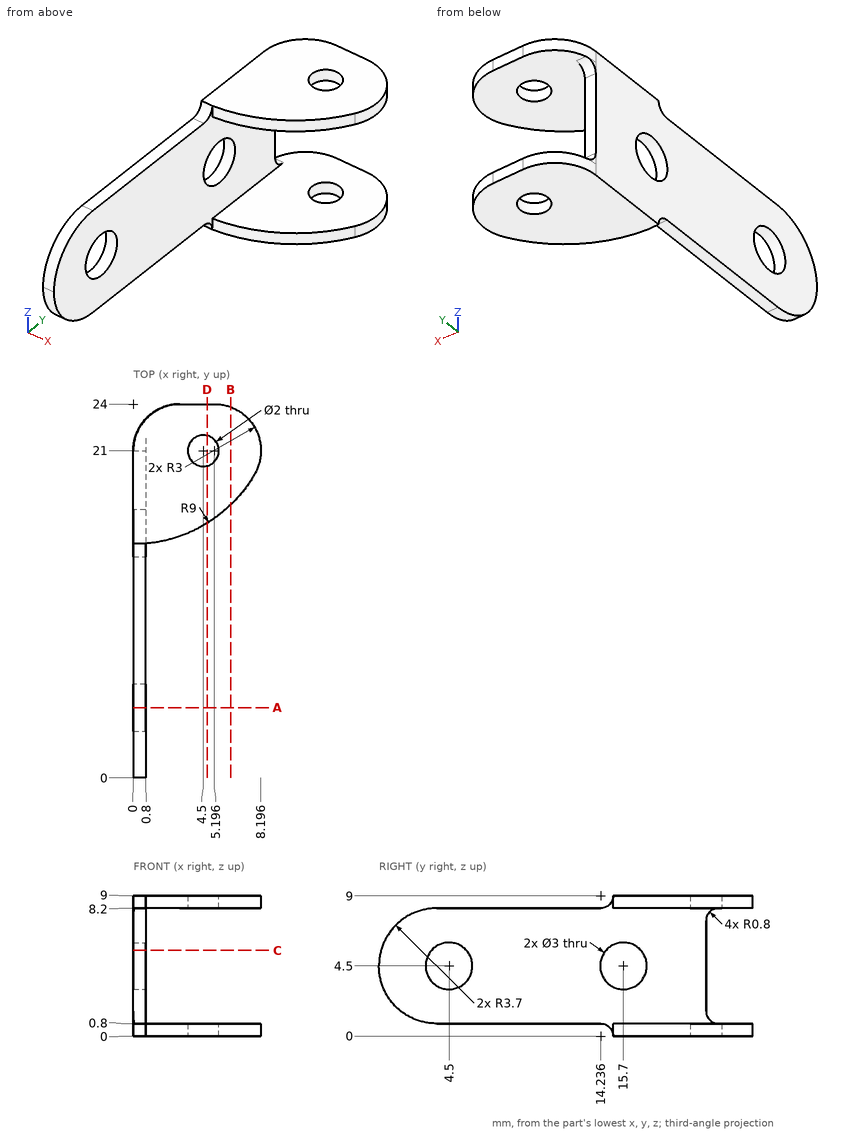
Here's the drawing with two shaded views (mm, measured from the low corner). I have some questions. Coordinates: 2 decimals unless noted, no trailing zeros. Order: outer loops, then holes, each group sorted by start corner. A loop starts at its lowest first (then second) coordinate and runs counter-clockwise, first axis right, second up. Notation, with made-up numbers: (-14, -12) - (22, -12) arc R14 ccw to (22, 5) - close; hole circle Ø8 at (38.25, -13). An arc over 180 degrees is marked (long way). Answer in a Markdown table with one row per item. Add a question column.
(1) If we section it at C-C, the plane z = 5.5: Please give me the cut outline in (x, y).
(2) I need wall thicknesses on L1, parallel to Z at x = 0.5, y = 15.7; L2, parallel to Z at x = 5.75, y = 20.25; L3, parallel to X at y = 14, z = 5. Which ranges of each line are inside material? Lowest first, please.
(3) Will this pin go through, and if not, where does the flat tip stop? pin 1 (1.8 mm diameter, centred on y = 15.7, z = 4.5, fed in from +X).
(4) If we section it at A-A, the plane y = 4.5: Please give me the cut outline in (x, z).
(5) If we section it at B-B, the plane x = 6.25: Please give me the cut outline in (y, z).
(6) If we section it at D-D, the plane x = 4.75: Please give me the cut outline in (y, z) (1 decimal).
Results are:
| question | item | result |
|---|---|---|
| 1 | outline | (0, 0.14) - (0.8, 0.14) - (0.8, 3.38) - (0, 3.38) - close; (0, 5.62) - (0.8, 5.62) - (0.8, 14.58) - (0, 14.58) - close; (0, 16.82) - (0.8, 16.82) - (0.8, 21) - (0, 21) - close |
| 2 | L1 | z = 0 to 3, 6 to 9 |
| 2 | L2 | z = 0 to 0.8, 8.2 to 9 |
| 2 | L3 | x = 0 to 0.8 |
| 3 | pin 1 | passes through |
| 4 | outline | (0, 0.8) - (0.8, 0.8) - (0.8, 3) - (0, 3) - close; (0, 6) - (0.8, 6) - (0.8, 8.2) - (0, 8.2) - close |
| 5 | outline | (17.52, 0) - (23.81, 0) - (23.81, 0.8) - (17.52, 0.8) - close; (17.52, 8.2) - (23.81, 8.2) - (23.81, 9) - (17.52, 9) - close |
| 6 | outline | (16.4, 0) - (20, 0) - (20, 0.8) - (16.4, 0.8) - close; (16.4, 8.2) - (20, 8.2) - (20, 9) - (16.4, 9) - close; (22, 0) - (24, 0) - (24, 0.8) - (22, 0.8) - close; (22, 8.2) - (24, 8.2) - (24, 9) - (22, 9) - close |
